```python
from build123d import *

# Parameters (mm, degrees)
F1_DEPTH      = 40
F1_DEPTH_BACK = 40


with BuildPart() as f1:
    # F0 (on Front) → F1 (new body, two sides)
    with BuildSketch(Plane.XZ) as f1_sk:
        with BuildLine():
            Line((18.4, 4.9), (0, 4.9))
            Line((0, 4.9), (-18.4, 4.9))
            ThreePointArc((-18.4, 4.9), (-18.753553, 4.753553), (-18.9, 4.4))
            Line((-18.9, 4.4), (-18.9, 2.9))
            Line((-18.9, 2.9), (-16, 0))
            Line((-16, 0), (-18.9, -2.9))
            Line((-18.9, -2.9), (-18.9, -4.4))
            ThreePointArc((-18.9, -4.4), (-18.753553, -4.753553), (-18.4, -4.9))
            Line((-18.4, -4.9), (0, -4.9))
            Line((0, -4.9), (18.4, -4.9))
            ThreePointArc((18.4, -4.9), (18.753553, -4.753553), (18.9, -4.4))
            Line((18.9, -4.4), (18.9, -2.9))
            Line((18.9, -2.9), (16, 0))
            Line((16, 0), (18.9, 2.9))
            Line((18.9, 2.9), (18.9, 4.4))
            ThreePointArc((18.9, 4.4), (18.753553, 4.753553), (18.4, 4.9))
        make_face()
    extrude(amount=F1_DEPTH)
    extrude(f1_sk.sketch, amount=-F1_DEPTH_BACK)


solid = f1.part
```
The listing builds one solid part. Answer for the finished solid, in the listing's coordinates (mm). A direction names the side the tool comes from. Coordinates: 2 decimals unless noted, no trailing zeros. Write each loop counter-clockwise with the first axis right and the second up, starting at its lowest first coordinate (ties: lowest second). Pieces come first, ordered by that corner, then holes. Notation, with made-up numbers: M 11,-11.75 L 52,-11.75 A33 ccw 52,23.25 Z; hole C -10.75,-15.75 d5. An arc over 180 degrees is marked long. Use a Markdown table: item, result. Add a question column.
1. Which of the six approach directions +Z, -Z, +X, -X, +Y, -Y give full straight-line access (tool end or side, diameter ignored) to faces 1 (the flat face through (-17, -1, 1)), 2 (the flat face through (17, -1, 1)), 3 (the flat face through (18.9, -1, -4))?
2. Straight lines are drawn through the part: line 1 along Z through (x, y) = (-17, 17.5); line 2 along X through (y, z) = (-10.5, 0); line 3 along X through (y, z) = (27.5, 0.75). For each, find the intervals that lie inside material, in ascending order. Write a range as [from, to].
3. Section B-B (z = 1.25) is taken. Give the vertices of the cut face in (x, y).
4. Given P1, Ø2, axis at y = 20.5, z = -2.5, coming from the -X side, flat-ended and moving along its own axis, determine where the tip first touches the part or whether it passes through.
5. Section A-A (y = -14.5) is taken. Give the vertices of the cut face in (x, z).
Data:
| question | item | result |
|---|---|---|
| 1 | face 1 | -X, +Y, -Y |
| 1 | face 2 | +X, +Y, -Y |
| 1 | face 3 | +Z, -Z, +X, +Y, -Y |
| 2 | line 1 | z = [-4.9, -1], [1, 4.9] |
| 2 | line 2 | x = [-16, 16] |
| 2 | line 3 | x = [-16.75, 16.75] |
| 3 | outline | M -17.25,-40 L 17.25,-40 L 17.25,40 L -17.25,40 Z |
| 4 | P1 | stops at x = -18.9 |
| 5 | outline | M -18.9,-4.4 A0.5 ccw -18.4,-4.9 L 18.4,-4.9 A0.5 ccw 18.9,-4.4 L 18.9,-2.9 L 16,0 L 18.9,2.9 L 18.9,4.4 A0.5 ccw 18.4,4.9 L -18.4,4.9 A0.5 ccw -18.9,4.4 L -18.9,2.9 L -16,0 L -18.9,-2.9 Z |
